Part model, mm, in its own coordinate system. Round coordinates to 2 decimals unless told otherwise and drop trailing zeros. Loops run counter-clockwise (first coordinate to the right, second up) from the corner with the lowest first, then second, coordinate; pieces in that order, holes last. Notation, with made-up numbers: (37.25, -9.5) -> (42.25, -9.5) arc R24 ccw to (42.25, 21.5) -> close; hole circle Ø5 at (-9.75, 72). An arc over 180 degrees is marked (long way). Answer as a JSON object with one key per item and string values. Group by question number.
Autodesk Inventor part; units mm, degrees
ref_plane "YZ Plane" through (0, 0, 0) normal (1, 0, 0) x (0, 1, 0)
ref_plane "XZ Plane" through (0, 0, 0) normal (0, 1, 0) x (-1, 0, 0)
ref_plane "XY Plane" through (0, 0, 0) normal (0, 0, 1) x (1, 0, 0)
sketch "Skizze1" plane through (0, 0, 0) normal (0, 0, 1) x (1, 0, 0)
  circle A0 centre (0, 0) radius 4
  dimension "d0" = 8
extrude "Extrusion1" add sketch "Skizze1" along normal blind 15
chamfer "Fase1" distance 0.5 angle 45 2 edges at (-4, 0, 15) (-4, 0, 0)
sketch "Skizze2" plane through (0, 0, 15) normal (0, 0, 1) x (1, 0, 0)
  circle A0 centre (0, 0) radius 3.5
hole "Bohrung1" at (0, 0, 15) direction (0, 0, -1) diameter 3.242 depth 10 tip angle 118
properties part number "1_0204_008"
Item 1: Band-saw the part on A-A, the plane z = 9.75. List the corners of the cut face in (x, y), plus the area to 3 significant figures.
Item 2: Drop a flat-ended pin along its axis: pin 1 Ø4 at (y, z) = (-0.5, 11) entering from -X. Give the stop position or say it passes through.
Item 3: Two-plate mould, pull along X, no slides. Class faces 1 (the face through (1.438, -0.748, 9.93)), 2 (the face through (-0.275, 0.061, 4.195)), 3 (the face through (1, -2, 15)), 4 (the face through (-0.867, 3.905, 7.402)): pulls with the +X half, pulls with the -X half, needs draft (parallel to the pull), parting line crosses it, or undercut.
Item 4: Drill centre lines: line 1 (Y direction, x = 0, z = 12.25); line 2 (Y direction, x = -1, z = 1); line 3 (Y direction, x = -1, z = 7.5). Where is each one in solid material? Low to high.
Item 5: Band-saw the part on B-B, the plane z = 1.5. List the corners of the cut face in (x, y).
Entries:
{
 "1": {"outline": "circle Ø8 at (0, 0); hole circle Ø3.24 at (0, 0)", "area": "42.0 mm²"},
 "2": {"pin 1": "x = -4"},
 "3": {"face 1": "undercut", "face 2": "undercut", "face 3": "needs draft", "face 4": "parting line crosses it"},
 "4": {"line 1": "-4 to -1.62, 1.62 to 4", "line 2": "-3.87 to 3.87", "line 3": "-3.87 to -1.28, 1.28 to 3.87"},
 "5": {"outline": "circle Ø8 at (0, 0)"}
}
